```python
from build123d import *

# Parameters (mm, degrees)
F0_W     = 100
F0_H     = 90
F1_DEPTH = 1
F2_W     = 89.622498
F2_H     = 14
F3_DEPTH = 5
F4_W     = 89.818385
F4_H     = 42.9
F5_DEPTH = 5


with BuildPart() as f1:
    # F0 (on Top) → F1 (new body)
    with BuildSketch(Plane.XY):
        with Locations((-50, 45)):
            Rectangle(F0_W, F0_H)
    extrude(amount=F1_DEPTH)

    # F2 (on Top) → F3 (join)
    with BuildSketch(Plane.XY):
        with Locations((-50.005771, 77.865734)):
            Rectangle(F2_W, F2_H)
    extrude(amount=F3_DEPTH)

    # F4 (on Top) → F5 (join)
    with BuildSketch(Plane.XY):
        with Locations((-50.002643, 30.7011)):
            Rectangle(F4_W, F4_H)
    extrude(amount=F5_DEPTH)


solid = f1.part
```
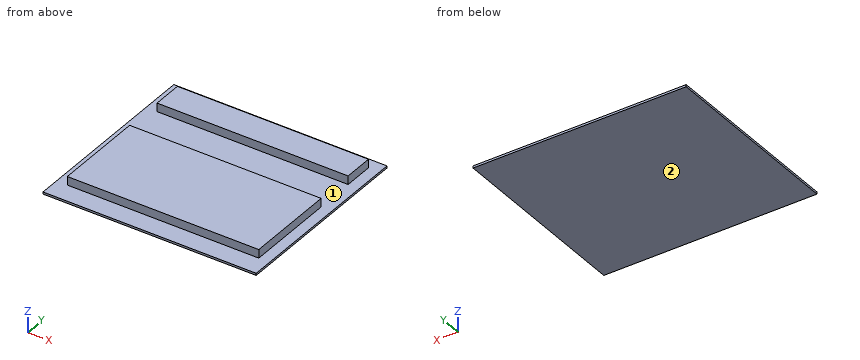
Model file for the job. Use its own axes, mm. Face numbers are marked on the shaded views. Give positions to 0.01 mm unless a question says otherwise; leave off trailing zeros. Write each loop counter-clockwise with the first axis right and the second up, starting at its lowest first coordinate (ties: lowest second). Pieces come first, ordered by that corner, then holes. Notation, with made-up numbers: (52.25, 78) -> (78.25, 78) arc R34 cw to (78.25, 108) -> close; hole circle Ø6 at (46, 48.25). An arc over 180 degrees is marked (long way). Use CSV: the item, a comma, the result in double quotes. Start each with the question number.
1) Pin check, flat tips, straight feed: P1, Ø2, axis at x = -38.5, z = 3.5, coming from the +Y side; P2, Ø1, axis at x = -12, y = 34.5, coming from the -Z side; P3, Ø1.2, axis at y = 34.5, z = 2, coming from the +X side; P4, Ø2, axis at y = 39.5, z = 3, coming from the -X side. Stop position of each tip, or through.
2) Two-plate mould, pull along Y, no slides. Class the marked faces 1 and 2: released by +Y, released by -Y, zero draft, split by the parting line, or undercut.
3) Cut at D-D on y = 72.5. List the corners of the cut face in (x, z), plus the area to 3 significant figures.
4) Cut at C-C on x = -8. List the corners of the cut face in (y, z).
5) Drill centre lines: L1, parallel to Y at x = -9, z = 3; L2, parallel to X at y = 36, z = 1.15; L3, parallel to Z at x = -5, y = 35.5. Where is each one in solid material? Low to high.
6) Cut at B-B on y = 26. List the corners of the cut face in (x, z).
7) Cut at A-A on z = 3.45. List the corners of the cut face in (x, y).
Final values:
1,P1,"stops at y = 84.87"
1,P2,"stops at z = 0"
1,P3,"stops at x = -5.09"
1,P4,"stops at x = -94.91"
2,face 1,"undercut"
2,face 2,"zero draft"
3,outline,"(-100, 0) -> (0, 0) -> (0, 1) -> (-5.19, 1) -> (-5.19, 5) -> (-94.82, 5) -> (-94.82, 1) -> (-100, 1) -> close"
3,area,"458 mm2"
4,outline,"(0, 0) -> (90, 0) -> (90, 1) -> (84.87, 1) -> (84.87, 5) -> (70.87, 5) -> (70.87, 1) -> (52.15, 1) -> (52.15, 5) -> (9.25, 5) -> (9.25, 1) -> (0, 1) -> close"
5,L1,"y = 9.25 to 52.15, 70.87 to 84.87"
5,L2,"x = -94.91 to -5.09"
5,L3,"z = 0 to 1"
6,outline,"(-100, 0) -> (0, 0) -> (0, 1) -> (-5.09, 1) -> (-5.09, 5) -> (-94.91, 5) -> (-94.91, 1) -> (-100, 1) -> close"
7,outline,"(-94.91, 9.25) -> (-5.09, 9.25) -> (-5.09, 52.15) -> (-94.91, 52.15) -> close; (-94.82, 70.87) -> (-5.19, 70.87) -> (-5.19, 84.87) -> (-94.82, 84.87) -> close"
